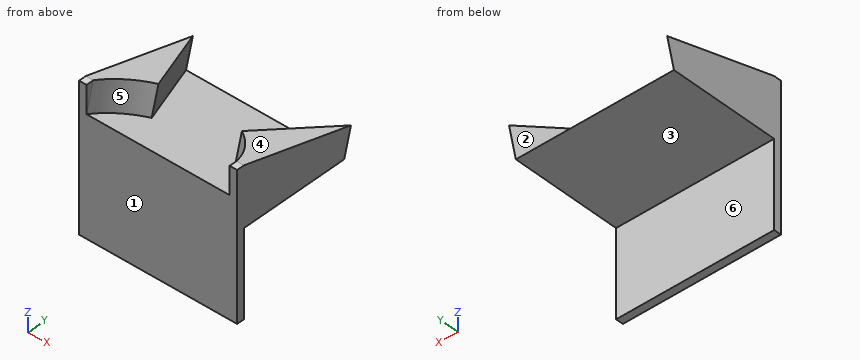
from build123d import *

# Parameters (mm, degrees)
F1_DEPTH = 5
F2_ANGLE = -15
F4_DEPTH = 27.4701582612
F5_W     = 27.4701582612
F5_H     = 15
F6_DEPTH = 1.3
F7_W     = 1.3
F7_H     = 4.8296291314


with BuildPart() as f1:
    # F0 (on Top) → F1 (new body)
    with BuildSketch(Plane.XY):
        with BuildLine():
            ThreePointArc((-12.4350791306, 0), (-10.4463192127, 3.9472350356), (-7.25, 7))
            Line((-7.25, 7), (-13.7350791306, 21.2054114289))
            Line((-13.7350791306, 21.2054114289), (-13.7350791306, 0))
            Line((-13.7350791306, 0), (-12.4350791306, 0))
        make_face()
    extrude(amount=F1_DEPTH)


with BuildPart() as f1b:
    # F0 (on Top) → F1, piece 2 (new body)
    with BuildSketch(Plane.XY):
        with BuildLine():
            Line((13.7350791306, 0), (13.7350791306, 21.2054114289))
            Line((13.7350791306, 21.2054114289), (7.25, 7))
            ThreePointArc((7.25, 7), (10.4463192127, 3.9472350356), (12.4350791306, 0))
            Line((12.4350791306, 0), (13.7350791306, 0))
        make_face()
    extrude(amount=F1_DEPTH)


with BuildPart() as f1_1:
    # F2: moved
    add(f1.part.rotate(Axis((0.65, 0, 0), (1, 0, 0)), F2_ANGLE))



with BuildPart() as f1b_1:
    # F2: moved
    add(f1b.part.rotate(Axis((0.65, 0, 0), (1, 0, 0)), F2_ANGLE))


with BuildPart() as f1_2:
    add(f1_1.part)

    add(f1b_1.part)  # F4 merges F1b
    # F3 (on face) → F4 (join, through all)
    with BuildSketch(Plane.YZ.offset(13.7350791306)):
        Polygon((20.4828545563, -5.488364337), (0, 0), (0, -5.488364337), align=None)
    extrude(amount=-F4_DEPTH)

    # F5 (on face) → F6 (join)
    with BuildSketch(Plane.XZ):
        with Locations((0, -12.988364337)):
            Rectangle(F5_W, F5_H)
    extrude(amount=-F6_DEPTH)

    # F7 (on face) → F8 (join, up to the next surface of F1)
    with BuildSketch(Plane.XZ):
        with Locations((-13.0850791306, 2.4148145657)):
            Rectangle(F7_W, F7_H)
        with Locations((13.0850791306, 2.4148145657)):
            Rectangle(F7_W, F7_H)
    extrude(until=Until.NEXT, dir=(0, 1, 0))


solid = f1_2.part
Input: part model. Units: mm. Frame: model coordinates. Face numbers are marked on the shaded views. A direction names the side the tool comes from. Give positions to 0.01 mm unless a question says otherwise; leave off trailing zeros. Write each loop counter-clockwise with the first axis right and the second up, starting at its lowest first coordinate (ties: lowest second). Pieces come first, ordered by that corner, then holes. Notation, with made-up numbers: M 18.5,-4.5 L 34.5,-4.5 A6 cw 34.5,0.5 Z; hole C 41,-23.5 d3. An arc over 180 degrees is marked long. Use one line per item in the form item = value.
1. Mould query, pull axis Z, two halves, no side actions, for the marked faces 1, 2 and 3. Classes: released by +Z, released by -Z, zero draft, split by the parting line, or undercut.
Outcome:
face_1 = zero draft
face_2 = undercut
face_3 = released by -Z
2. Cut plane D-D on x = 8.75. Return loops of the section in (y, z), and give its area (3 significant figures).
Outcome:
outline = M 0,-20.49 L 1.3,-20.49 L 1.3,-5.49 L 20.48,-5.49 L 9.94,-2.66 L 11.23,2.17 L 6.92,3.32 L 5.63,-1.51 L 0,0 Z
area = 98.0 mm²
3. Cut plane B-B on y = 10.75. Return loops of the section in (x, z), and give its area (3 significant figures).
Outcome:
outline = M -13.74,-5.49 L 13.74,-5.49 L 13.74,2.3 L 8.52,2.3 L 9.14,-2.88 L -9.14,-2.88 L -8.52,2.3 L -13.74,2.3 Z
area = 122 mm²
4. Cut plane C-C on z = -14. Return loops of the section in (x, y), and give its area (3 significant figures).
Outcome:
outline = M -13.74,0 L 13.74,0 L 13.74,1.3 L -13.74,1.3 Z
area = 35.7 mm²
5. Reachability of the marked faces 4, 5 and 6 from +Z, -Z, +X, -X, +Y, -Y: full face, straight path, thin tool, end or side. Return the list, or none.
Outcome:
face_4 = +Z, +X, -X, +Y
face_5 = +Z
face_6 = -Z, +X, -X, +Y
6. First-contact query: P1, Ø6, axis at x = 10, y = 15, coming from the -Z side; P2, Ø3, axis at x = 4.5, y = 3, coming from the +Z side; P3, Ø1, axis at x = 3, y = 16, coming from the +Z side; P4, Ø4, axis at x = 3, z = 0.5, coming from the -Y side. Flat tips, straight axial feed; report the tip coordinate or a pass-through.
Outcome:
P1 = -5.49
P2 = -0.4
P3 = -4.15
P4 = 0
7. Cut plane A-A on x = -6.5. Return loops of the section in (y, z), and give its area (3 significant figures).
Outcome:
outline = M 0,-20.49 L 1.3,-20.49 L 1.3,-5.49 L 20.48,-5.49 L 0,0 Z
area = 75.7 mm²
8. Ray query, L1, parallel to Y at x = 3.75, z = -7.5; L2, parallel to X at y = 8, z = 3; L3, parallel to X at y = 21, z = -0.75. Return the intervals inside material, ascending.
Outcome:
L1 = 0 to 1.3
L2 = -13.74 to -7.32, 7.32 to 13.74
L3 = -13.74 to -13.4, 13.4 to 13.74
